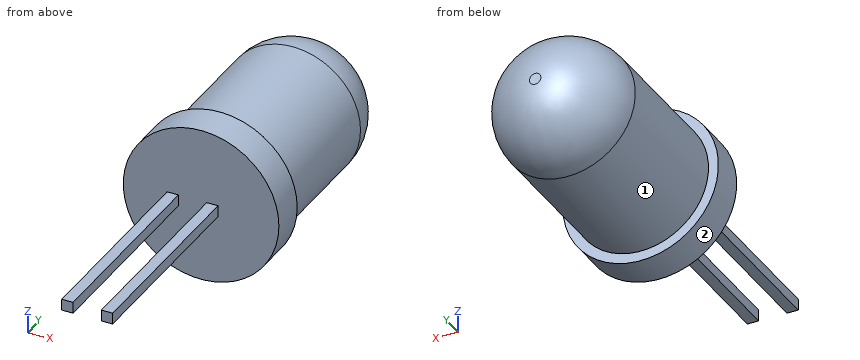
```python
from build123d import *

# Parameters (mm, degrees)
SKETCH1_R           = 2.75
BOSS_EXTRUDE1_DEPTH = 1.25
SKETCH2_R           = 2.4
BOSS_EXTRUDE2_DEPTH = 7.2
FILLET1_R           = 2.2
SKETCH3_W           = 0.4
SKETCH3_H           = 0.4
BOSS_EXTRUDE3_DEPTH = 7.2


with BuildPart() as part:
    # Sketch1 → Boss-Extrude1 (new body)
    with BuildSketch(Plane(origin=(0, 0, 0), x_dir=(1, 0, 0), z_dir=(0, 1, 0))):
        Circle(SKETCH1_R)
    extrude(amount=BOSS_EXTRUDE1_DEPTH)

    # Sketch2 → Boss-Extrude2 (add)
    with BuildSketch(Plane(origin=(0, 1.25, 0), x_dir=(1, 0, 0), z_dir=(0, 1, 0))):
        Circle(SKETCH2_R)
    extrude(amount=BOSS_EXTRUDE2_DEPTH)

    # Fillet1
    fillet1_edges = [part.edges().sort_by_distance(p)[0] for p in [
        (-2.4, 8.45, 0),
    ]]
    fillet(fillet1_edges, radius=FILLET1_R)

    # Sketch3 → Boss-Extrude3 (add)
    with BuildSketch(Plane.XZ):
        with Locations((-1, -0.060309903)):
            Rectangle(SKETCH3_W, SKETCH3_H)
    boss_extrude3 = extrude(amount=BOSS_EXTRUDE3_DEPTH)

    # Mirror2: Boss-Extrude3 across plane
    add(boss_extrude3.mirror(Plane(origin=(-0.3, 0, 0), x_dir=(0, 0, 1), z_dir=(1, 0, 0))))


solid = part.part
```
The model under review builds one solid part; all positions refer to its coordinate system, in mm. Face numbers are marked on the shaded views. A direction names the side the tool comes from. Round coordinates to 2 decimals unless told otherwise and drop trailing zeros. Order: outer loops, then holes, each group sorted by start corner. A loop starts at its lowest first (then second) coordinate and runs counter-clockwise, first axis right, second up.
Item 1: Machinability: for the marked faces 1 and 2, which of the approach directions +Z, -Z, +X, -X, +Y, -Y give a long, thin tool a straight path to every point of the face, cutting with its end or side? Answer none if there is none.
Working result:
face 1: +Y
face 2: +Y, -Y
Item 2: To check wall thickness, follow probe 1 along X at (y, z) = (7.5, 0.45); probe 2 along Y at (x, z) = (-0.05, 1.65); probe 3 along X at (y, z) = (6.75, 1.9). State the ranges of each line that lie inside material, in increasing order.
Working result:
probe 1: x = -1.96 to 1.96
probe 2: y = 0 to 7.9
probe 3: x = -1.37 to 1.37
Item 3: For pin 1 (1 mm diameter, centred on y = -3, z = 0, fed in from +X); pin 2 (2 mm diameter, centred on x = -1.5, z = -2, fed in from +Y); pin 3 (1 mm diameter, centred on x = 0, y = 5, fed in from -Z), all flat-tipped, find the tip position at first contact; note any pin that passes through.
Working result:
pin 1: stops at x = 0.6
pin 2: stops at y = 8.02
pin 3: stops at z = -2.4
Item 4: Add section B-B, the plane y = 2.25. State the section outline as (x, z) points, and give its area (3 significant figures).
Working result:
outline: circle Ø4.8 at (0, 0)
area: 18.1 mm2
Item 5: Add section A-A, the plane y = -2.75. State the section outline as (x, z) points.
Working result:
outline: (-1.2, -0.26) - (-0.8, -0.26) - (-0.8, 0.14) - (-1.2, 0.14) - close; (0.2, -0.26) - (0.6, -0.26) - (0.6, 0.14) - (0.2, 0.14) - close
